Verification items for the finished model (mm, model axes). Give positions to 0.01 mm unless a question says otherwise; leave off trailing zeros. Order: outer loops, then holes, each group sorted by start corner. A loop starts at its lowest first (then second) coordinate and runs counter-clockwise, first axis right, second up. Notation, with made-up numbers: (21.25, 54) - (64.25, 54) arc R26 cw to (64.25, 76) - close; hole circle Ø1 at (49.25, -25.5). An arc over 180 degrees is marked (long way). Answer as a JSON object with one key per item and string values.
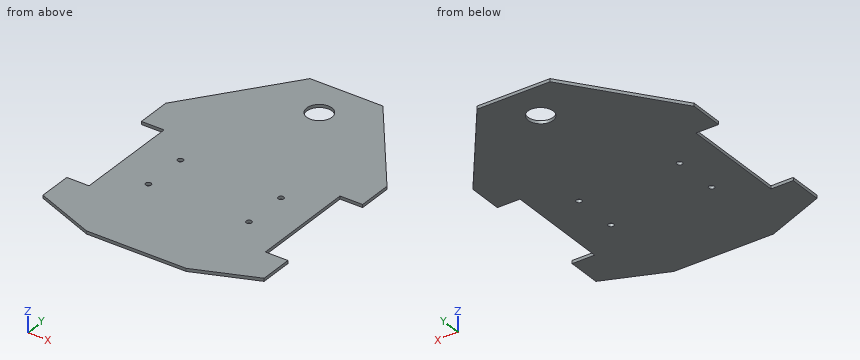
```python
from build123d import *

# Parameters (mm, degrees)
SKETCH1_R           = 1.1
BOSS_EXTRUDE1_DEPTH = 1.2
SKETCH2_R           = 5
CUT_EXTRUDE1_DEPTH  = 74.610053661


with BuildPart() as part:
    # Sketch1 → Boss-Extrude1 (new body)
    with BuildSketch(Plane.XY):
        Polygon((-19.807417596, -59), (-44, -49.322967039), (-44, -36), (-35.109892996, -36), (-35, 6), (-44, 6), (-44, 19.666666667), (-14.5, 59), (14.5, 59), (44, 19.666666667), (44, 6), (35, 6), (35, -36), (44, -36), (44, -49.322967039), (19.807417596, -59), align=None)
        with Locations((-20, -6)):
            Circle(SKETCH1_R, mode=Mode.SUBTRACT)
        with Locations((-20, -24)):
            Circle(SKETCH1_R, mode=Mode.SUBTRACT)
        with Locations((20, -6)):
            Circle(SKETCH1_R, mode=Mode.SUBTRACT)
        with Locations((20, -24)):
            Circle(SKETCH1_R, mode=Mode.SUBTRACT)
    extrude(amount=BOSS_EXTRUDE1_DEPTH)

    # Sketch2 → Cut-Extrude1 (cut, through all)
    with BuildSketch(Plane.XY.offset(1.2)):
        with Locations((0, 43.808911543)):
            Circle(SKETCH2_R)
    extrude(amount=-CUT_EXTRUDE1_DEPTH, mode=Mode.SUBTRACT)


solid = part.part
```
(1) Section check B-B (z = 0.75). Record the cut outline in (x, y).
Computed values:
{"outline": "(-44, -49.32) - (-19.81, -59) - (19.81, -59) - (44, -49.32) - (44, -36) - (35, -36) - (35, 6) - (44, 6) - (44, 19.67) - (14.5, 59) - (-14.5, 59) - (-44, 19.67) - (-44, 6) - (-35, 6) - (-35.11, -36) - (-44, -36) - close; hole circle Ø2.2 at (-20, -24); hole circle Ø2.2 at (-20, -6); hole circle Ø10 at (0, 43.81); hole circle Ø2.2 at (20, -24); hole circle Ø2.2 at (20, -6)"}
(2) Section check D-D (x = 38.5). Record the cut outline in (y, z), then the cut area to 3 significant figures.
Computed values:
{"outline": "(-51.52, 0) - (-36, 0) - (-36, 1.2) - (-51.52, 1.2) - close; (6, 0) - (27, 0) - (27, 1.2) - (6, 1.2) - close", "area": "43.8 mm²"}
(3) Gauge pin test, flat end, axial feed: pin 1 Ø1.3 at (x, y) = (20, -6) entering from -Z. Record the tip position at first contact, or that the pin passes through.
Computed values:
{"pin 1": "passes through"}
(4) Section check A-A (x = 0). Record the cut outline in (y, z), then the cut area to 3 significant figures.
Computed values:
{"outline": "(-59, 0) - (38.81, 0) - (38.81, 1.2) - (-59, 1.2) - close; (48.81, 0) - (59, 0) - (59, 1.2) - (48.81, 1.2) - close", "area": "130 mm²"}
(5) Section check C-C (y = 22). Record the cut outline in (x, z), then the cut area to 3 significant figures.
Computed values:
{"outline": "(-42.25, 0) - (42.25, 0) - (42.25, 1.2) - (-42.25, 1.2) - close", "area": "101 mm²"}
(6) Material ranges on line 1 along Y through (x, z) = (20, 0.5); line 2 along X through (y, z) = (40.5, 1.15) (3 decimals); line 3 along X through (y, z) = (4.5, 0.45), recorded low to high. Write a range as [from, to].
Computed values:
{"line 1": "y = [-58.92, -25.1], [-22.9, -7.1], [-4.9, 51.67]", "line 2": "x = [-28.375, -3.748], [3.748, 28.375]", "line 3": "x = [-35, 35]"}
